from build123d import *

# Parameters (mm, degrees)
BOSS_EXTRUDE1_DEPTH      = 1.5
BOSS_EXTRUDE1_DEPTH_BACK = 1.5
SKETCH1_R                = 20
SKETCH1_R_2              = 2.475
SKETCH2_W                = 12
SKETCH2_H                = 2.85
CUT_EXTRUDE1_DEPTH       = 29.442925307
CIRPATTERN1_COUNT        = 8


with BuildPart() as part:
    # Sketch1 → Boss-Extrude1 (new, two sides: drawn at the far end of the back side and taken through both)
    with BuildSketch(Plane(origin=(0, 0, 0), x_dir=(1, 0, 0), z_dir=(0, 1, 0)).offset(-BOSS_EXTRUDE1_DEPTH_BACK)):
        with Locations(Location((0, 0, 0), (0, 0, 270))):
            Circle(SKETCH1_R)
        with Locations(Location((0, 0, 0), (0, 0, 270))):
            Circle(SKETCH1_R_2, mode=Mode.SUBTRACT)
    extrude(amount=BOSS_EXTRUDE1_DEPTH + BOSS_EXTRUDE1_DEPTH_BACK)

    # Sketch2 → Cut-Extrude1 (cut, through all)
    with BuildSketch(Plane(origin=(0, 1.5, 0), x_dir=(1, 0, 0), z_dir=(0, 1, 0))):
        with Locations((20, 0)):
            Rectangle(SKETCH2_W, SKETCH2_H)
    cut_extrude1 = extrude(amount=-CUT_EXTRUDE1_DEPTH, mode=Mode.SUBTRACT)

    # CirPattern1: Cut-Extrude1 ×8 about axis
    cirpattern1_axis = Axis((0, 0, 0), (0, 1, 0))
    for i in range(1, CIRPATTERN1_COUNT):
        add(cut_extrude1.rotate(cirpattern1_axis, i * 360 / CIRPATTERN1_COUNT), mode=Mode.SUBTRACT)


solid = part.part
Could you check a few things on this model? Use its own coordinates, in mm. A direction names the side the tool comes from. Round coordinates to 2 decimals unless told otherwise and drop trailing zeros. Loops run counter-clockwise (first coordinate to the right, second up) from the corner with the lowest first, then second, coordinate; pieces in that order, holes last. Notation, with made-up numbers: (10.5, 66) - (43.5, 66) arc R30 cw to (43.5, 105) - close; hole circle Ø4 at (-9.75, 7). An arc over 180 degrees is marked (long way). Write item = value, one per line.
1) If we mould it in two halves opening along Z, with no side actions, what happens to faces 1 (the flat face through (0, 0, -14)), 2 (the flat face through (-1.425, 0, 17)), 3 (the flat face through (17, 0, 1.425))? For each: pulls with the +Z half, pulls with the -Z half, needs draft (parallel to the pull), parting line crosses it, or undercut.
Computed:
face_1 = pulls with the -Z half
face_2 = needs draft
face_3 = undercut
2) I'm going to push flat-ended pins straight in: P1, Ø1.4, axis at x = 0, y = 0.5, coming from the +Z side; P2, Ø1.5, axis at x = -18, y = 0.5, coming from the +Z side; P3, Ø1.5, axis at x = 18, y = 0.5, coming from the -Z side. Where does each tip first touch, or does it pass through?
Computed:
P1 = 14
P2 = 10.12
P3 = -10.12
3) Imagine slicing it at C-C (z = 0). Please give me the cut outline in (x, y) (3 decimals).
Computed:
outline = (-14, -1.5) - (-2.475, -1.5) - (-2.475, 1.5) - (-14, 1.5) - close; (2.475, -1.5) - (14, -1.5) - (14, 1.5) - (2.475, 1.5) - close
4) Imagine slicing it at B-B (x = 0). Please give me the cut outline in (y, z) (3 decimals), and give its area (4 significant figures).
Computed:
outline = (-1.5, -14) - (1.5, -14) - (1.5, -2.475) - (-1.5, -2.475) - close; (-1.5, 2.475) - (1.5, 2.475) - (1.5, 14) - (-1.5, 14) - close
area = 69.15 mm2
5) I need wall thicknesses on line 1 along X through (y, z) = (0.8, 0) (3 decimals); line 2 along X through (y, z) = (0.75, 12); line 3 along X through (y, z) = (1.3, -12.5). Which ranges of each line are inside material? Lowest first, please. Write a range as from..to.
Computed:
line_1 = -14..-2.475, 2.475..14
line_2 = -16..-14.02, -9.98..9.98, 14.02..16
line_3 = -15.61..-14.52, -10.48..10.48, 14.52..15.61
6) On a 3-axis mill with a long thin cutter (end or side, diameter ignored), from which of +Z, -Z, +X, -X, +Y, -Y can I reach the whole of each face in a straight line? I mean faces 4 (the flat face through (-14, 0, 0)), 5 (the flat face through (12.981, 0.021, 10.966)), 6 (the flat face through (-1.425, 0, -17)). Say none if no direction works.
Computed:
face_4 = -X, +Y, -Y
face_5 = +Y, -Y
face_6 = -Z, +Y, -Y
7) Imagine slicing it at D-D (x = -10). Please give me the cut outline in (y, z), and give its area (3 significant figures).
Computed:
outline = (-1.5, -17.32) - (1.5, -17.32) - (1.5, -12.02) - (-1.5, -12.02) - close; (-1.5, -9.8) - (1.5, -9.8) - (1.5, 9.8) - (-1.5, 9.8) - close; (-1.5, 12.02) - (1.5, 12.02) - (1.5, 17.32) - (-1.5, 17.32) - close
area = 90.6 mm2
